Read the model definition and answer for the solid it produces. Units are mm, in the model's axes. A direction names the side the tool comes from. Coordinates: 2 decimals unless noted, no trailing zeros. Order: outer loops, then holes, each group sorted by start corner. A loop starts at its lowest first (then second) coordinate and runs counter-clockwise, first axis right, second up. Notation, with made-up numbers: (24.5, 73) -> (48.5, 73) arc R16 ccw to (48.5, 80) -> close; hole circle Ø11 at (58, 85.25). An arc over 180 degrees is marked (long way). Answer in a Markdown table with one row per item.
from build123d import *

# Parameters (mm, degrees)
SKETCH1_R           = 2.1
BOSS_EXTRUDE1_DEPTH = 8
CUT_EXTRUDE1_REACH  = 63.082
SKETCH2_R           = 1.65


with BuildPart() as part:
    # Sketch1 → Boss-Extrude1 (new body)
    with BuildSketch(Plane.XY):
        with BuildLine():
            Line((-14.353967242, 72.5), (5, 72.5))
            Line((5, 72.5), (5, 80))
            Line((5, 80), (-19.131994198, 80))
            Line((-19.131994198, 80), (-38.637128513, 38.171104477))
            ThreePointArc((-38.637128513, 38.171104477), (-38.911873787, 35.832206145), (-37.737913805, 33.790699757))
            ThreePointArc((-37.737913805, 33.790699757), (-11.724148086, 20.607586106), (17.400101197, 22.120396774))
            ThreePointArc((17.400101197, 22.120396774), (19.816194151, 26.841360112), (15.095230814, 29.257453067))
            ThreePointArc((15.095230814, 29.257453067), (-8.815701312, 27.678006068), (-30.628506806, 37.599137276))
            Line((-30.628506806, 37.599137276), (-14.353967242, 72.5))
        make_face()
        with Locations((0, 76)):
            Circle(SKETCH1_R, mode=Mode.SUBTRACT)
        with Locations((-30.947084331, 33.134292287)):
            Circle(SKETCH1_R, mode=Mode.SUBTRACT)
        with Locations((-35.238474323, 36.58628597)):
            Circle(SKETCH1_R, mode=Mode.SUBTRACT)
        with Locations((16.247666005, 25.68892492)):
            Circle(SKETCH1_R, mode=Mode.SUBTRACT)
        with Locations((10.932992292, 24.273211913)):
            Circle(SKETCH1_R, mode=Mode.SUBTRACT)
        with Locations((5.5, 23.417294418)):
            Circle(SKETCH1_R, mode=Mode.SUBTRACT)
        with Locations((-26.319869018, 30.147460036)):
            Circle(SKETCH1_R, mode=Mode.SUBTRACT)
        with Locations((-16.261912507, 25.693527972)):
            Circle(SKETCH1_R, mode=Mode.SUBTRACT)
        with Locations((-10.940316211, 24.274760441)):
            Circle(SKETCH1_R, mode=Mode.SUBTRACT)
        with Locations((-21.407041065, 27.658201118)):
            Circle(SKETCH1_R, mode=Mode.SUBTRACT)
        with Locations((-5.5, 23.417294418)):
            Circle(SKETCH1_R, mode=Mode.SUBTRACT)
        with Locations((0, 23.130434783)):
            Circle(SKETCH1_R, mode=Mode.SUBTRACT)
    extrude(amount=BOSS_EXTRUDE1_DEPTH)

    # Sketch2 → Cut-Extrude1 (cut, up to next)
    with BuildSketch(Plane(origin=(-46.356679233, 21.616474533, 0), x_dir=(0, 0, 1), z_dir=(-0.906307787, 0.422618262, 0)), mode=Mode.PRIVATE) as cut_extrude1_sk1:
        with Locations((4, 55.04255297)):
            Circle(SKETCH2_R)
    cut_extrude1_tool1 = extrude(cut_extrude1_sk1.sketch, amount=-CUT_EXTRUDE1_REACH, mode=Mode.PRIVATE) & part.part
    add(cut_extrude1_tool1.solids().sort_by_distance((-23.094691, 71.501969, 4))[0], mode=Mode.SUBTRACT)
    # Sketch2 → Cut-Extrude1 (cut, up to next)
    with BuildSketch(Plane(origin=(-46.356679233, 21.616474533, 0), x_dir=(0, 0, 1), z_dir=(-0.906307787, 0.422618262, 0)), mode=Mode.PRIVATE) as cut_extrude1_sk2:
        with Locations((4, 27.64255297)):
            Circle(SKETCH2_R)
    cut_extrude1_tool2 = extrude(cut_extrude1_sk2.sketch, amount=-CUT_EXTRUDE1_REACH, mode=Mode.PRIVATE) & part.part
    add(cut_extrude1_tool2.solids().sort_by_distance((-34.674432, 46.669136, 4))[0], mode=Mode.SUBTRACT)


solid = part.part
Q1. The part is cut by section C-C (z = 6.5). Give the number of separate pieces and of enclosed holes in the cut face, then the cut area to 3 significant figures.
Outcome:
| item | result |
|---|---|
| separate pieces | 1 |
| enclosed holes | 12 |
| area | 759 mm² |
Q2. Consider line 1 (Y direction, x = 0, z = 4.5); line 2 (Y direction, x = -23, z = 0.5); line 3 (Y direction, x = -21.5, z = 1.5). Determine where each line is inside the solid, lowest interval first.
Outcome:
| item | result |
|---|---|
| line 1 | 19.38 to 21.03, 25.23 to 26.88, 72.5 to 73.9, 78.1 to 80 |
| line 2 | 24.26 to 26.29, 29.03 to 32.6, 53.96 to 71.71 |
| line 3 | 23.62 to 25.56, 29.76 to 31.84, 57.18 to 74.92 |
Q3. The part is cut by section D-D (x = 0). Write down the section's boundary in (y, z), then the cut area to 3 significant figures.
Outcome:
| item | result |
|---|---|
| outline | (19.38, 0) -> (21.03, 0) -> (21.03, 8) -> (19.38, 8) -> close; (25.23, 0) -> (26.88, 0) -> (26.88, 8) -> (25.23, 8) -> close; (72.5, 0) -> (73.9, 0) -> (73.9, 8) -> (72.5, 8) -> close; (78.1, 0) -> (80, 0) -> (80, 8) -> (78.1, 8) -> close |
| area | 52.8 mm² |
Q4. The part is cut by section A-A (x = -6.5). Write down the section's boundary in (y, z).
Outcome:
| item | result |
|---|---|
| outline | (19.75, 0) -> (21.57, 0) -> (21.57, 8) -> (19.75, 8) -> close; (25.26, 0) -> (27.31, 0) -> (27.31, 8) -> (25.26, 8) -> close; (72.5, 0) -> (80, 0) -> (80, 8) -> (72.5, 8) -> close |
Q5. For a pull along Y with two mould halves and no side action, classify faces 4 (the face through (-16.535, 27.776, 3.944)), 5 (the face through (-27, 50, 0)), 6 (the face through (-12.128, 20.695, 3.944)), 7 (the face through (-7, 80, 4)) as pulls with the +Y half, pulls with the -Y half, needs draft (parallel to the pull), parting line crosses it, or undercut.
Outcome:
| item | result |
|---|---|
| face 4 | undercut |
| face 5 | needs draft |
| face 6 | pulls with the -Y half |
| face 7 | pulls with the +Y half |
Q6. For faces 1 (the face through (5, 76, 4)), 2 (the face through (-22.605, 54.805, 3.944)), 3 (the face through (-8.482, 27.618, 3.944)), determine the directions among +Z, -Z, +X, -X, +Y, -Y from which every point of the face is accessible in a straight line to the end or side of a thin tool.
Outcome:
| item | result |
|---|---|
| face 1 | +Z, -Z, +X, +Y |
| face 2 | +Z, -Z, +X |
| face 3 | +Z, -Z |
Q7. The part is cut by section B-B (y = 76). Write down the section's boundary in (x, z), then the cut area to 3 significant figures.
Outcome:
| item | result |
|---|---|
| outline | (-21, 0) -> (-2.1, 0) -> (-2.1, 8) -> (-21, 8) -> close; (2.1, 0) -> (5, 0) -> (5, 8) -> (2.1, 8) -> close |
| area | 174 mm² |
Q8. Given pin 1 (1.5 mm diameter, centred on x = -32, z = 4, fed in from +Y); pin 2 (2 mm diameter, centred on y = 48.5, z = 6.5, fed in from +X); pin 3 (2 mm diameter, centred on y = 77.5, z = 2.5, fed in from +X), each flat-ended and moving along its own axis, determine where each tip first touches the part or whether it passes through.
Outcome:
| item | result |
|---|---|
| pin 1 | y = 54.01 |
| pin 2 | x = -25.08 |
| pin 3 | x = 5 |
